Input: part model. Units: mm. Frame: model coordinates. A direction names the side the tool comes from. Coordinates: 2 decimals unless noted, no trailing zeros. Order: outer loops, then holes, each group sorted by start corner. A loop starts at its lowest first (then second) coordinate and runs counter-clockwise, first axis right, second up. Notation, with made-up numbers: M 84.5,72.5 L 138.5,72.5 A13 ccw 138.5,78.5 Z; hole C -11.75,51 d6. An arc over 180 degrees is marked long. One line per item, written item: value.
```python
from build123d import *

# Parameters (mm, degrees)
EXTRUDE_1_DEPTH     = 15
CUT_EXTRUDE_1_DEPTH = 80.214897589
SKETCH_3_R          = 40
EXTRUDE_2_DEPTH     = 240
SKETCH_4_R          = 35.5
EXTRUDE_3_DEPTH     = 4
SKETCH_5_R          = 37.5
EXTRUDE_4_DEPTH     = 28
CHAMFER_1_SIZE      = 2


with BuildPart() as part:
    # 草图1 → 凸台-拉伸1 (new body)
    with BuildSketch(Plane.XY):
        Polygon((-27.5, 47.631397208), (-47.631397208, 27.5), (-55, 0), (-47.631397208, -27.5), (-27.5, -47.631397208), (0, -55), (27.5, -47.631397208), (47.631397208, -27.5), (55, 0), (47.631397208, 27.5), (27.5, 47.631397208), (0, 55), align=None)
    extrude(amount=EXTRUDE_1_DEPTH)

    # 草图2 → 切除-拉伸1 (cut, through all)
    with BuildSketch(Plane.XY.offset(15)):
        Polygon((-47.631397208, 27.5), (-47.631397208, -27.5), (-55, 0), align=None)
        Polygon((47.631397208, 27.5), (47.631397208, -27.5), (55, 0), align=None)
    extrude(amount=-CUT_EXTRUDE_1_DEPTH, mode=Mode.SUBTRACT)

    # 草图3 → 凸台-拉伸2 (add)
    with BuildSketch(Plane(origin=(0, 0, 0), x_dir=(-1, 0, 0), z_dir=(0, 0, -1))):
        with Locations(Location((0, 0, 0), (0, 0, 180))):
            Circle(SKETCH_3_R)
    extrude(amount=EXTRUDE_2_DEPTH)

    # 草图4 → 凸台-拉伸3 (add)
    with BuildSketch(Plane(origin=(0, 0, -240), x_dir=(-1, 0, 0), z_dir=(0, 0, -1))):
        Circle(SKETCH_4_R)
    extrude(amount=EXTRUDE_3_DEPTH)

    # 草图5 → 凸台-拉伸4 (add)
    with BuildSketch(Plane(origin=(0, 0, -244), x_dir=(-1, 0, 0), z_dir=(0, 0, -1))):
        Circle(SKETCH_5_R)
    extrude(amount=EXTRUDE_4_DEPTH)

    # 倒角1
    chamfer_1_edges = [part.edges().sort_by_distance(p)[0] for p in [
        (13.75, 51.315698604, 0),
        (37.565698604, 37.565698604, 0),
        (37.565698604, -37.565698604, 0),
        (13.75, -51.315698604, 0),
        (-13.75, -51.315698604, 0),
        (-37.565698604, -37.565698604, 0),
        (-37.565698604, 37.565698604, 0),
        (-13.75, 51.315698604, 0),
        (-37.565698604, -37.565698604, 15),
        (-13.75, -51.315698604, 15),
        (13.75, -51.315698604, 15),
        (37.565698604, -37.565698604, 15),
        (37.565698604, 37.565698604, 15),
        (-47.631397208, 0, 0),
        (13.75, 51.315698604, 15),
        (-47.631397208, 0, 15),
        (-13.75, 51.315698604, 15),
        (-40, 0, -240),
        (37.5, 0, -272),
        (-37.565698604, 37.565698604, 15),
    ]]
    chamfer(chamfer_1_edges, length=CHAMFER_1_SIZE)


solid = part.part
```
(1) Cut plane A-A on y = 0. Output: boundary loops of the cut face in (x, z).
Data:
outline: M -47.63,2 L -45.63,0 L -40,0 L -40,-238 L -38,-240 L -35.5,-240 L -35.5,-244 L -37.5,-244 L -37.5,-270 L -35.5,-272 L 35.5,-272 L 37.5,-270 L 37.5,-244 L 35.5,-244 L 35.5,-240 L 38,-240 L 40,-238 L 40,0 L 47.63,0 L 47.63,15 L -45.63,15 L -47.63,13 Z
(2) Access query for faces 1 (the flat face through (-11, -34, -240)), 2 (the cylindrical face through (-39.96, -1.76, -117.33)), 3 (the flat face through (0, 1, 15)). Directions: +Z, -Z, +X, -X, +Y, -Y. A direction counts if a zero-diameter tool reaches every point of the face in a straight line with its end or side. Return the directions, or none.
Data:
face 1: none
face 2: -Z
face 3: +Z, +X, -X, +Y, -Y
(3) Draft query along Z for faces 4 (the flat face through (-33, -14, -244)), 5 (the flat face through (37.71, 37.42, 7.42)), 6 (the flat face through (37.71, 35.99, 14.01)). Return one class per face: released by +Z, released by -Z, zero draft, split by the parting line, or undercut.
Data:
face 4: undercut
face 5: zero draft
face 6: released by +Z
(4) First-contact query: pin 1 (8 mm diameter, centred on x = -21, z = -43.5, fed in from -Y); pin 2 (5 mm diameter, centred on x = 12, z = -221, fed in from -Y); pin 3 (2 mm diameter, centred on x = 23.5, y = 29.5, fed in from -Z). Flat tips, straight axial feed; report the tip coordinate or a pass-through.
Data:
pin 1: stops at y = -36.21
pin 2: stops at y = -38.86
pin 3: stops at z = -270.78
(5) Cut plane B-B on z = -146.5. Output: boundary loops of the cut face in (x, y), plus the area to 3 significant figures.
Data:
outline: C 0,0 d80
area: 5,030 mm2
(6) Ray query, line 1 (Z direction, x = 22, y = 41); line 2 (Y direction, x = 5, z = -5.5); line 3 (X direction, y = 23.5, z = -49). Return the intervals inside material, ascending. Write a range as from..to.
Data:
line 1: z = 0..15
line 2: y = -39.69..39.69
line 3: x = -32.37..32.37
